```python
from build123d import *

# Parameters (mm, degrees)
F0_R     = 1.65
F1_DEPTH = 1.5
F2_R     = 1


# Not quite as in the source:
# - ends of sketch curves that miss each other by under 0.0002 mm in the source are joined


with BuildPart() as f1:
    # F0 (on Top) → F1 (new body)
    with BuildSketch(Plane.XY):
        with BuildLine():
            ThreePointArc((19.6082164698, -11.4503983868), (13.339608, 1.2499996959), (19.608215987, 13.9503980169))
            ThreePointArc((19.608215987, 13.9503980169), (19.8967236619, 14.3015730303), (20.000004, 14.744172))
            Line((20.000004, 14.744172), (20.000004, 17.25))
            ThreePointArc((20.000004, 17.25), (19.8535573906, 17.6035533906), (19.500004, 17.75))
            Line((19.500004, 17.75), (14.500004, 17.75))
            ThreePointArc((14.500004, 17.75), (14.1464506094, 17.6035533906), (14.000004, 17.25))
            Line((14.000004, 17.25), (14.000004, 16.25))
            ThreePointArc((14.000004, 16.25), (13.4441182966, 15.5255556337), (12.6004849604, 15.8749999771))
            ThreePointArc((12.6004849604, 15.8749999771), (12.3259659886, 16.1495190594), (11.950966, 16.25))
            Line((11.950966, 16.25), (-11.950958, 16.25))
            ThreePointArc((-11.950958, 16.25), (-12.3259579886, 16.1495190594), (-12.6004770396, 15.8750000229))
            ThreePointArc((-12.6004770396, 15.8750000229), (-13.4441102966, 15.5255556337), (-13.999996, 16.25))
            Line((-13.999996, 16.25), (-13.999996, 17.25))
            ThreePointArc((-13.999996, 17.25), (-14.1464426094, 17.6035533906), (-14.499996, 17.75))
            Line((-14.499996, 17.75), (-19.499996, 17.75))
            ThreePointArc((-19.499996, 17.75), (-19.8535493906, 17.6035533906), (-19.999996, 17.25))
            Line((-19.999996, 17.25), (-19.999996, 14.744172))
            ThreePointArc((-19.999996, 14.744172), (-19.8967156619, 14.3015730303), (-19.6082083041, 13.9503976031))
            ThreePointArc((-19.6082083041, 13.9503976031), (-13.3396, 1.2499996959), (-19.6082084698, -11.4503983868))
            ThreePointArc((-19.6082084698, -11.4503983868), (-19.8967227718, -11.8015703601), (-20.000004, -12.244173))
            Line((-20.000004, -12.244173), (-19.999996, -17.25))
            ThreePointArc((-19.999996, -17.25), (-19.8535493906, -17.6035533906), (-19.499996, -17.75))
            Line((-19.499996, -17.75), (-14.499996, -17.75))
            ThreePointArc((-14.499996, -17.75), (-14.1464426094, -17.6035533906), (-13.999996, -17.25))
            Line((-13.999996, -17.25), (-13.999996, -13.75))
            ThreePointArc((-13.999996, -13.75), (-13.4441102966, -13.0255556337), (-12.6004769604, -13.3749999771))
            ThreePointArc((-12.6004769604, -13.3749999771), (-12.3259579886, -13.6495190594), (-11.950958, -13.75))
            Line((-11.950958, -13.75), (11.950966, -13.75))
            ThreePointArc((11.950966, -13.75), (12.3259659886, -13.6495190594), (12.6004850396, -13.3750000229))
            ThreePointArc((12.6004850396, -13.3750000229), (13.4441182966, -13.0255556337), (14.000004, -13.75))
            Line((14.000004, -13.75), (14.000004, -17.25))
            ThreePointArc((14.000004, -17.25), (14.1464506094, -17.6035533906), (14.500004, -17.75))
            Line((14.500004, -17.75), (19.500004, -17.75))
            ThreePointArc((19.500004, -17.75), (19.8535573906, -17.6035533906), (20.000004, -17.25))
            Line((20.000004, -17.25), (20.000004, -12.244173))
            ThreePointArc((20.000004, -12.244173), (19.8967236619, -11.8015740303), (19.6082164698, -11.4503983868))
        make_face()
        with Locations((-4.8728769961, 1.25)):
            Circle(F0_R, mode=Mode.SUBTRACT)
        with BuildLine():
            ThreePointArc((-0.3045548123, -4.6981452929), (1.8543964627, -2.0656887385), (2.6271230039, 1.25))
            ThreePointArc((2.6271230039, 1.25), (1.938751938, 4.3887435806), (0, 6.9513217574))
            Line((0, 6.9513217574), (0, 10.550810168))
            ThreePointArc((0, 10.550810168), (4.1108641083, 6.6852916914), (5.6271230039, 1.25))
            ThreePointArc((5.6271230039, 1.25), (4.1108641083, -4.1852916914), (0, -8.050810168))
            Line((0, -8.050810168), (-0.3045548123, -4.6981452929))
        make_face(mode=Mode.SUBTRACT)
    extrude(amount=F1_DEPTH)

    # F2
    f2_edges = [f1.edges().sort_by_distance(p)[0] for p in [
        (0, 10.55081, 0.75),
        (-0.304555, -4.698145, 0.75),
        (0, -8.05081, 0.75),
        (0, 6.951322, 0.75),
    ]]
    fillet(f2_edges, radius=F2_R)


solid = f1.part
```
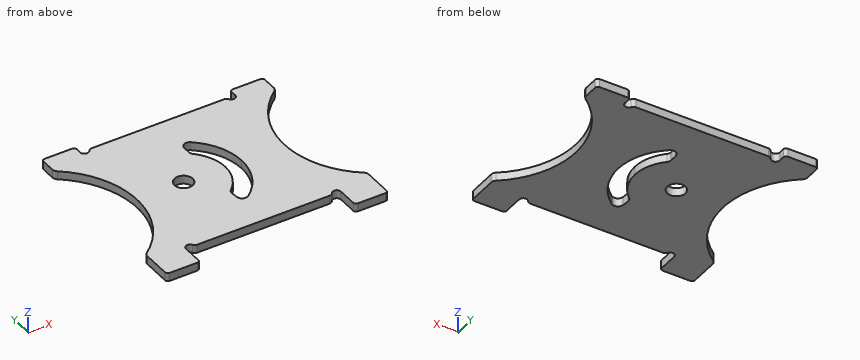
Design review of the part built by this model. Coordinates are the model's own, in mm. Give positions to 0.01 mm unless a question says otherwise; leave off trailing zeros. Loops run counter-clockwise (first coordinate to the right, second up) from the corner with the lowest first, then second, coordinate; pieces in that order, holes last. Notation, with made-up numbers: M 39.25,-22.5 L 84.25,-22.5 A12 cw 84.25,-13.5 Z; hole C -1.5,-39.75 d3. An arc over 180 degrees is marked long. Return JSON: item names as keys, results as strings. Group by question number.
Item 1: For probe 1 along X at (y, z) = (0, 0.85); probe 2 along X at (y, z) = (5.5, 0.75); probe 3 along Y at (x, z) = (16, 0.5), list the stretches that pass through material, from the lowest coordinate up.
Item 2: We need section C-C (z = 0.95). Give the number of separate pieces and of enclosed holes in the cut face, and give its area (3 significant figures).
Item 3: We need section D-D (y = 13). Give the boundary of the cut face in (x, z), and give its area (3 significant figures).
Item 4: We need section A-A (x = 15). Give the boundary of the cut face in (y, z), and give its area (3 significant figures).
Item 5: We need section B-B (y = 5). Give the boundary of the cut face in (x, z), and give its area (3 significant figures).
Output:
{
 "1": {"probe 1": "x = -13.39 to -5.95, -3.8 to 2.52, 5.55 to 13.39", "probe 2": "x = -13.91 to 1.31, 4.73 to 13.91", "probe 3": "y = -17.75 to -7.58, 10.08 to 17.75"},
 "2": {"separate pieces": "1", "enclosed holes": "2", "area": "958 mm^2"},
 "3": {"outline": "M -18.48,0 L 18.48,0 L 18.48,1.5 L -18.48,1.5 Z", "area": "55.4 mm^2"},
 "4": {"outline": "M -17.75,0 L -5.85,0 L -5.85,1.5 L -17.75,1.5 Z; M 8.35,0 L 17.75,0 L 17.75,1.5 L 8.35,1.5 Z", "area": "32.0 mm^2"},
 "5": {"outline": "M -13.79,0 L 1.62,0 L 1.62,1.5 L -13.79,1.5 Z; M 4.93,0 L 13.79,0 L 13.79,1.5 L 4.93,1.5 Z", "area": "36.4 mm^2"}
}
